Verification items for this drawing (mm, ordinates from the low corner). Round coordinates to 2 decimals unless told otherwise and drop trailing zeros. Write each loop counter-clockwise with the first axis right and the second up, starting at its lowest first coordinate (ties: lowest second). Pieces come first, ordered by that corner, then holes. Notation, with made-up numbers: M -30.75,70 L 1.25,70 A13 ccw 1.25,88 Z; hole C -2,9 d1. An arc over 180 degrees is marked long. One line per question, with ' | ' between items. Start each with the question number.
Q1. Cross-section at A-A (z = 43.5). Record the boundary of the cut face in (x, y) (3 decimals), then the cut area to 3 significant figures.
Q2. Cross-section at C-C (y = 2.15). Record the boundary of the cut face in (x, z).
Q3. Cross-section at B-B (x = 12.5). Record the boundary of the cut face in (y, z) (3 decimals), then the cut area to 3 significant figures.
Q4. Cross-section at D-D (x = 46). Record the boundary of the cut face in (y, z) (3 decimals), then the cut area to 3 significant figures.
Q5. Thickness scan on line 1 along X through (y, z) = (1.8, 80); line 2 along X through (y, z) = (2.95, 41); line 3 along Z through (x, y) = (28, 1.7). Record the ranges inside material, lowest first. Write a range as from..to.
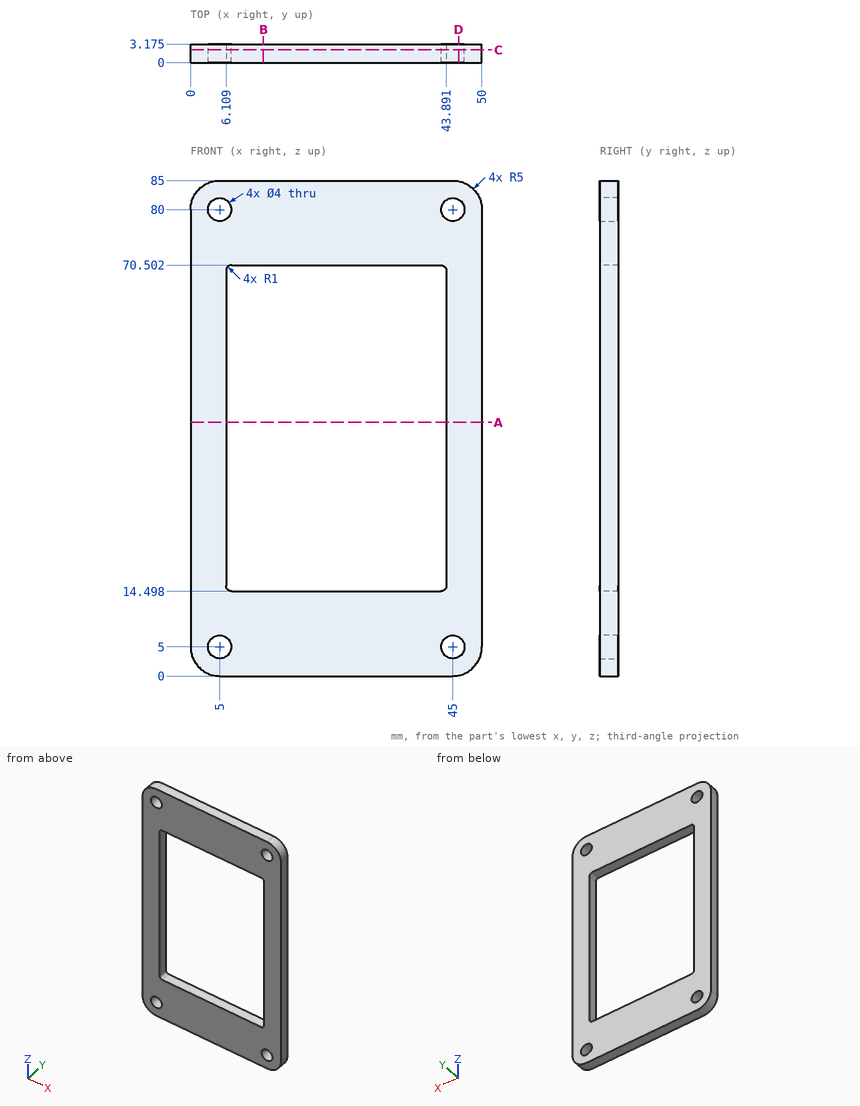
Determined:
1) outline: M 0,0 L 6.109,0 L 6.109,3.175 L 0,3.175 Z; M 43.891,0 L 50,0 L 50,3.175 L 43.891,3.175 Z | area: 38.8 mm²
2) outline: M 0,5 A5 ccw 5,0 L 45,0 A5 ccw 50,5 L 50,80 A5 ccw 45,85 L 5,85 A5 ccw 0,80 Z; hole C 5,5 d4; hole C 5,80 d4; hole M 6.11,15.5 A1 ccw 7.11,14.5 L 42.89,14.5 A1 ccw 43.89,15.5 L 43.89,69.5 A1 ccw 42.89,70.5 L 7.11,70.5 A1 ccw 6.11,69.5 Z; hole C 45,5 d4; hole C 45,80 d4
3) outline: M 0,0 L 3.175,0 L 3.175,14.498 L 0,14.498 Z; M 0,70.502 L 3.175,70.502 L 3.175,85 L 0,85 Z | area: 92.1 mm²
4) outline: M 0,0.101 L 3.175,0.101 L 3.175,3.268 L 0,3.268 Z; M 0,6.732 L 3.175,6.732 L 3.175,78.268 L 0,78.268 Z; M 0,81.732 L 3.175,81.732 L 3.175,84.899 L 0,84.899 Z | area: 247 mm²
5) line 1: x = 0..3, 7..43, 47..50 | line 2: x = 0..6.11, 43.89..50 | line 3: z = 0..14.5, 70.5..85
